Source: CAD feature listing. Evaluate the final solid. Frame: model axes, mm. Face numbers are marked on the shaded views. Round coordinates to 2 decimals unless told otherwise and drop trailing zeros. Order: outer loops, then holes, each group sorted by start corner. A loop starts at its lowest first (then second) coordinate and runs counter-clockwise, first axis right, second up. Notation, with made-up numbers: (52, 33.25) -> (57, 33.25) arc R37 cw to (57, 71.25) -> close; hole circle Ø5 at (16.5, 26.25). An arc over 180 degrees is marked (long way). Use a Markdown table: item, result. Add a question column.
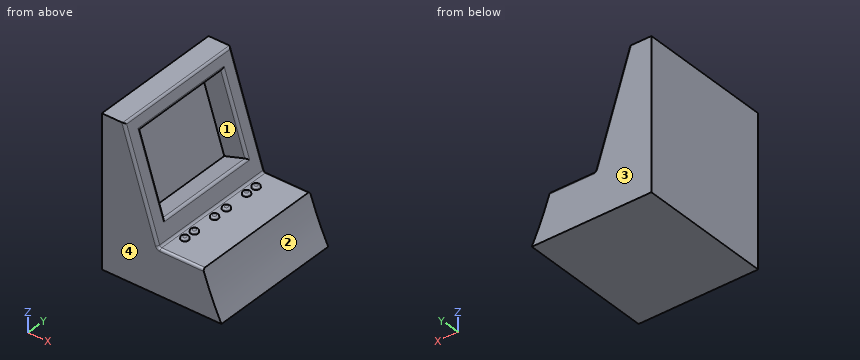
```python
from build123d import *

# Parameters (mm, degrees)
F1_DEPTH = 450
F2_W     = 347
F2_H     = 261
F3_DEPTH = 80
F4_F1_R  = 8
F4_F2_R  = 8
F5_R     = 12.5
F6_DEPTH = 7


# Not quite as in the source:
# - a fillet or chamfer that OpenCascade refuses, or shapes differently, is made with other operations: its cross-section is extruded or revolved along the edge and cut away or added


with BuildPart() as f1:
    # F0 (on Front) → F1 (new body)
    with BuildSketch(Plane.XZ):
        with BuildLine():
            Line((-120.4737946391, 342.6808416843), (-195.4737946391, 342.6808416843))
            Line((-195.4737946391, 342.6808416843), (-195.4737946391, -157.3191583157))
            Line((-195.4737946391, -157.3191583157), (204.5262053609, -157.3191583157))
            ThreePointArc((204.5262053609, -157.3191583157), (171.3461744918, -83.3583725961), (143.2543578127, -7.3191583157))
            Line((143.2543578127, -7.3191583157), (-6.7456421873, -7.3191583157))
            Line((-6.7456421873, -7.3191583157), (-120.4737946391, 342.6808416843))
        make_face()
    extrude(amount=F1_DEPTH)

    # F2 (on face) → F3 (cut)
    with BuildSketch(Plane(origin=(-8.2525689762, 0, -2.681569779), x_dir=(0, 1, 0), z_dir=(0.951051518, 0, 0.3090323772))):
        with Locations((-225, 188.1374378125)):
            Rectangle(F2_W, F2_H)
    extrude(amount=-F3_DEPTH, mode=Mode.SUBTRACT)

    # F4: fillet of radius 8 on 8 edges, made by hand

    # F4_f1
    f4_f1_edges = [f1.edges().sort_by_distance(p)[0] for p in [
        (-6.7456421873, -225, -7.3191583157),
    ]]
    fillet(f4_f1_edges, radius=F4_F1_R)

    # F4_f2
    f4_f2_edges = [f1.edges().sort_by_distance(p)[0] for p in [
        (-64.5078037977, 0, 170.4447121755),
        (-64.5078037977, -450, 170.4447121755),
        (-120.4737946391, -225, 342.6808416843),
        (-66.3931286265, -398.5, 176.2468260396),
        (-106.7218538531, -225, 300.3590491347),
        (-66.3931286265, -51.5, 176.2468260396),
        (-26.0644034, -225, 52.1346029445),
        (-5.6356304889, -450, -5.791332299),
        (-5.6356304889, 0, -5.791332299),
    ]]
    fillet(f4_f2_edges, radius=F4_F2_R)

    # F5 (on face) → F6 (join)
    with BuildSketch(Plane.XY.offset(-7.3191583157)):
        with Locations((20.8874940872, -372.5)):
            Circle(F5_R)
        with Locations((20.8874940872, -332.5)):
            Circle(F5_R)
        with Locations((20.8874940872, -247.5)):
            Circle(F5_R)
        with Locations((20.8874940872, -197.5)):
            Circle(F5_R)
        with Locations((20.8874940872, -112.5)):
            Circle(F5_R)
        with Locations((20.8874940872, -72.5)):
            Circle(F5_R)
    extrude(amount=F6_DEPTH)

    # F7: fillet of radius 7 on 1 edges, made by hand

    # F7_s1 → F7_t2 (revolve, cut)
    with BuildSketch(Plane.XZ.offset(372.5)):
        with BuildLine():
            add(Edge.make_bspline(
                [(33.3874940872, -7.3191583157), (33.3874940872, -0.3191583157), (26.3874940872, -0.3191583157)],
                knots=[0, 0, 0, 1, 1, 1], degree=2, weights=[1, 2.3333333333, 1]))
            Line((26.3874940872, -0.3191583157), (33.3874940872, -0.3191583157))
            Line((33.3874940872, -0.3191583157), (33.3874940872, -7.3191583157))
        make_face()
    revolve(axis=Axis((20.8874940872, -372.5, -0.3191583157), (0, 0, 1)), mode=Mode.SUBTRACT)

    # F8: fillet of radius 7 on 5 edges, made by hand

    # F8_s1 → F8_t2 (revolve, cut)
    with BuildSketch(Plane.XZ.offset(332.5)):
        with BuildLine():
            add(Edge.make_bspline(
                [(33.3874940872, -7.3191583157), (33.3874940872, -0.3191583157), (26.3874940872, -0.3191583157)],
                knots=[0, 0, 0, 1, 1, 1], degree=2, weights=[1, 2.3333333333, 1]))
            Line((26.3874940872, -0.3191583157), (33.3874940872, -0.3191583157))
            Line((33.3874940872, -0.3191583157), (33.3874940872, -7.3191583157))
        make_face()
    revolve(axis=Axis((20.8874940872, -332.5, -0.3191583157), (0, 0, 1)), mode=Mode.SUBTRACT)

    # F8_s3 → F8_t4 (revolve, cut)
    with BuildSketch(Plane.XZ.offset(197.5)):
        with BuildLine():
            add(Edge.make_bspline(
                [(33.3874940872, -7.3191583157), (33.3874940872, -0.3191583157), (26.3874940872, -0.3191583157)],
                knots=[0, 0, 0, 1, 1, 1], degree=2, weights=[1, 2.3333333333, 1]))
            Line((26.3874940872, -0.3191583157), (33.3874940872, -0.3191583157))
            Line((33.3874940872, -0.3191583157), (33.3874940872, -7.3191583157))
        make_face()
    revolve(axis=Axis((20.8874940872, -197.5, -0.3191583157), (0, 0, 1)), mode=Mode.SUBTRACT)

    # F8_s5 → F8_t6 (revolve, cut)
    with BuildSketch(Plane.XZ.offset(247.5)):
        with BuildLine():
            add(Edge.make_bspline(
                [(33.3874940872, -7.3191583157), (33.3874940872, -0.3191583157), (26.3874940872, -0.3191583157)],
                knots=[0, 0, 0, 1, 1, 1], degree=2, weights=[1, 2.3333333333, 1]))
            Line((26.3874940872, -0.3191583157), (33.3874940872, -0.3191583157))
            Line((33.3874940872, -0.3191583157), (33.3874940872, -7.3191583157))
        make_face()
    revolve(axis=Axis((20.8874940872, -247.5, -0.3191583157), (0, 0, 1)), mode=Mode.SUBTRACT)

    # F8_s7 → F8_t8 (revolve, cut)
    with BuildSketch(Plane.XZ.offset(112.5)):
        with BuildLine():
            add(Edge.make_bspline(
                [(33.3874940872, -7.3191583157), (33.3874940872, -0.3191583157), (26.3874940872, -0.3191583157)],
                knots=[0, 0, 0, 1, 1, 1], degree=2, weights=[1, 2.3333333333, 1]))
            Line((26.3874940872, -0.3191583157), (33.3874940872, -0.3191583157))
            Line((33.3874940872, -0.3191583157), (33.3874940872, -7.3191583157))
        make_face()
    revolve(axis=Axis((20.8874940872, -112.5, -0.3191583157), (0, 0, 1)), mode=Mode.SUBTRACT)

    # F8_s9 → F8_t10 (revolve, cut)
    with BuildSketch(Plane.XZ.offset(72.5)):
        with BuildLine():
            add(Edge.make_bspline(
                [(33.3874940872, -7.3191583157), (33.3874940872, -0.3191583157), (26.3874940872, -0.3191583157)],
                knots=[0, 0, 0, 1, 1, 1], degree=2, weights=[1, 2.3333333333, 1]))
            Line((26.3874940872, -0.3191583157), (33.3874940872, -0.3191583157))
            Line((33.3874940872, -0.3191583157), (33.3874940872, -7.3191583157))
        make_face()
    revolve(axis=Axis((20.8874940872, -72.5, -0.3191583157), (0, 0, 1)), mode=Mode.SUBTRACT)


solid = f1.part
```
1) Section D-D on z = -74. Output: boundary loops of the cut face in (x, y).
2) Draft query along Y for the marked faces 1, 2, 3 and 4. Return one class per face: pulls with the +Y half, pulls with the -Y half, needs draft (parallel to the pull), parting line crosses it, or undercut.
3) Line query: probe 1 along Y at (x, z) = (-115.5, 279.5); probe 2 along Z at (x, y) = (78.5, -86); probe 3 along Z at (x, y) = (20.5, -340). Output: solid intervals per line, ascending. Write a range as from..to.
4) Section A-A on x = -158. Output: boundary loops of the cut face in (y, z), then the cut area to 3 significant figures.
5) Section B-B on x = 115. Output: boundary loops of the cut face in (y, z), then the cut area to 3 significant figures.
6) Section C-C on y = -168. Output: boundary loops of the cut face in (x, z), then the cut area to 3 significant figures.
7) First-contact query: pin 1 Ø3.5 at (x, y) = (20, -335) entering from +Z; pin 2 Ø4 at (y, z) = (-112, 57.5) entering from +X. Flat tips, straight axial feed; report the tip coordinate or a pass-through.
Conclusion:
| question | item | result |
|---|---|---|
| 1 | outline | (-195.47, -450) -> (167.57, -450) -> (167.57, 0) -> (-195.47, 0) -> close |
| 2 | face 1 | undercut |
| 2 | face 2 | needs draft |
| 2 | face 3 | pulls with the +Y half |
| 2 | face 4 | pulls with the -Y half |
| 3 | probe 1 | y = -450..-398.5, -51.5..0 |
| 3 | probe 2 | z = -157.32..-7.32 |
| 3 | probe 3 | z = -157.32..-0.36 |
| 4 | outline | (-450, -157.32) -> (0, -157.32) -> (0, 342.68) -> (-450, 342.68) -> close; hole (-398.5, 199.3) -> (-51.5, 199.3) -> (-51.5, 283.7) -> (-398.5, 283.7) -> close |
| 4 | area | 196,000 mm^2 |
| 5 | outline | (-450, -157.32) -> (0, -157.32) -> (0, -15.32) arc R8 ccw to (-8, -7.32) -> (-442, -7.32) arc R8 ccw to (-450, -15.32) -> close |
| 5 | area | 67,500 mm^2 |
| 6 | outline | (-195.47, -157.32) -> (204.53, -157.32) arc R1195.54 cw to (143.25, -7.32) -> (-0.93, -7.32) arc R8 cw to (-8.54, -1.79) -> (-23.59, 44.53) arc R8 ccw to (-33.67, 49.66) -> (-102.15, 27.41) -> (-182.81, 275.64) -> (-114.33, 297.89) arc R8 ccw to (-109.19, 307.97) -> (-118.68, 337.15) arc R8 ccw to (-126.29, 342.68) -> (-195.47, 342.68) -> close |
| 6 | area | 80,400 mm^2 |
| 7 | pin 1 | stops at z = -0.32 |
| 7 | pin 2 | stops at x = -111.28 |
